For this review, take the finished solid that the model builds, in its own axes (mm). Give positions to 0.01 mm unless a question says otherwise; leave off trailing zeros. Loops run counter-clockwise (first coordinate to the right, second up) from the corner with the lowest first, then second, coordinate; pieces in that order, holes last. Notation, with made-up numbers: (-28.75, 80) -> (-1.75, 80) arc R25 cw to (-1.75, 107) -> close; hole circle Ø9 at (83.5, -26). An arc over 180 degrees is marked (long way). One line per question, with ' | ' between items. Start each with the question number.
(1) Consider section A-A (y = 4). Write out the cut boundary in (x, z).
(2) Insertion check: P1, Ø2.5, axis at y = 0, z = 69.85, coming from the +X side. The pin has a flat end and moves straight along its axis. Give the tip position at first contact, or say it passes through.
(3) Wall thickness on probe 1 along Z at (x, y) = (-1.85, -4); probe 2 along Y at (x, z) = (-1.1, 3); probe 3 along Z at (x, y) = (-2.4, 30.5): over which ranges is each line inside the solid? List them lowest first.
(4) Consider section B-B (x = -1.15). Give the number of separate pieces and of enclosed holes in the cut face, and give its area (3 significant figures).
from build123d import *

# Parameters (mm, degrees)
SKETCH1_W                       = 279.4
SKETCH1_H                       = 76.2
BOSS_EXTRUDE1_DEPTH             = 3
SKETCH3_W                       = 3
SKETCH3_H                       = 15
CUT_EXTRUDE1_DEPTH              = 145.833352512
LPATTERN1_COUNT                 = 3
LPATTERN1_PITCH                 = 22.8
MIRROR1_COPY_1_SKETCH_W         = 3
MIRROR1_COPY_1_SKETCH_H         = 15
MIRROR1_COPY_1_DEPTH            = 145.833352512
MIRROR1_COPY_2_SKETCH_W         = 3
MIRROR1_COPY_2_SKETCH_H         = 15
MIRROR1_COPY_2_DEPTH            = 145.833352512
F_3_0MM_CLEARANCE_DOWEL_HOLE1_D = 3
SKETCH6_W                       = 3
SKETCH6_H                       = 7.8
CUT_EXTRUDE2_DEPTH              = 145.833352512
LPATTERN2_COUNT                 = 4
LPATTERN2_PITCH                 = 22.8
SKETCH7_W                       = 3
SKETCH7_H                       = 7.8
CUT_EXTRUDE3_DEPTH              = 10
LPATTERN3_COUNT                 = 2
LPATTERN3_PITCH                 = 22.8


with BuildPart() as part:
    # Sketch1 → Boss-Extrude1 (new body)
    with BuildSketch(Plane(origin=(0, 0, 0), x_dir=(0, 0, -1), z_dir=(1, 0, 0))):
        Rectangle(SKETCH1_W, SKETCH1_H)
    extrude(amount=-BOSS_EXTRUDE1_DEPTH)

    # Sketch3 → Cut-Extrude1 (cut, through all)
    with BuildSketch(Plane.ZY.offset(3)):
        with Locations((133.2, 22.8)):
            Rectangle(SKETCH3_W, SKETCH3_H)
    cut_extrude1 = extrude(amount=-CUT_EXTRUDE1_DEPTH, mode=Mode.SUBTRACT)

    # LPattern1: Cut-Extrude1 ×3
    with Locations(*[(0, -i * LPATTERN1_PITCH, 0) for i in range(1, LPATTERN1_COUNT)]):
        add(cut_extrude1, mode=Mode.SUBTRACT)

    # Mirror1: Cut-Extrude1 across plane
    add(cut_extrude1.mirror(Plane.XY), mode=Mode.SUBTRACT)

    # Mirror1 copy 1 sketch → Mirror1 copy 1 (cut, through all)
    with BuildSketch(Plane(origin=(-3, -22.8, 0), x_dir=(0, 0, -1), z_dir=(-1, 0, 0))):
        with Locations((133.2, -22.8)):
            Rectangle(MIRROR1_COPY_1_SKETCH_W, MIRROR1_COPY_1_SKETCH_H)
    extrude(amount=-MIRROR1_COPY_1_DEPTH, mode=Mode.SUBTRACT)

    # Mirror1 copy 2 sketch → Mirror1 copy 2 (cut, through all)
    with BuildSketch(Plane(origin=(-3, -45.6, 0), x_dir=(0, 0, -1), z_dir=(-1, 0, 0))):
        with Locations((133.2, -22.8)):
            Rectangle(MIRROR1_COPY_2_SKETCH_W, MIRROR1_COPY_2_SKETCH_H)
    extrude(amount=-MIRROR1_COPY_2_DEPTH, mode=Mode.SUBTRACT)

    # Ø3.0mm Clearance Dowel Hole1 (through all)
    with Locations(Plane.ZY.offset(3)):
        with Locations((69.85, 0)):
            Hole(F_3_0MM_CLEARANCE_DOWEL_HOLE1_D / 2)

    # Sketch6 → Cut-Extrude2 (cut, through all)
    with BuildSketch(Plane.ZY.offset(3)):
        with Locations((1.56, 34.2)):
            Rectangle(SKETCH6_W, SKETCH6_H)
    cut_extrude2 = extrude(amount=-CUT_EXTRUDE2_DEPTH, mode=Mode.SUBTRACT)

    # LPattern2: Cut-Extrude2 ×4
    with Locations(*[(0, -i * LPATTERN2_PITCH, 0) for i in range(1, LPATTERN2_COUNT)]):
        add(cut_extrude2, mode=Mode.SUBTRACT)

    # Sketch7 → Cut-Extrude3 (cut)
    with BuildSketch(Plane.ZY.offset(3)):
        with Locations((-80.2, 34.2)):
            Rectangle(SKETCH7_W, SKETCH7_H)
    cut_extrude3 = extrude(amount=-CUT_EXTRUDE3_DEPTH, mode=Mode.SUBTRACT)

    # LPattern3: Cut-Extrude3 ×2
    with Locations(*[(0, -i * LPATTERN3_PITCH, 0) for i in range(1, LPATTERN3_COUNT)]):
        add(cut_extrude3, mode=Mode.SUBTRACT)


solid = part.part
A:
1) outline: (-3, -139.7) -> (0, -139.7) -> (0, -134.7) -> (-3, -134.7) -> close; (-3, -131.7) -> (0, -131.7) -> (0, 131.7) -> (-3, 131.7) -> close; (-3, 134.7) -> (0, 134.7) -> (0, 139.7) -> (-3, 139.7) -> close
2) P1: passes through
3) probe 1: z = -139.7 to -134.7, -131.7 to 131.7, 134.7 to 139.7 | probe 2: y = -30.3 to -15.3, -7.5 to 7.5, 15.3 to 30.3 | probe 3: z = -139.7 to -81.7, -78.7 to 0.06, 3.06 to 139.7
4) separate pieces: 1 | enclosed holes: 10 | area: 20,900 mm^2
